Work out the finished part from the listing and answer in its coordinate system (mm). A direction names the side the tool comes from. Round coordinates to 2 decimals unless told otherwise and drop trailing zeros. Use one line per item in the form item = value. Start each with the question number.
Q1. Given P1, Ø10, axis at x = -24.5, y = -16, coming from the -Z side; P2, Ø12, axis at x = -12, z = -65.5, coming from the -Y side; P3, Ø2, axis at x = -10, z = -59, coming from the +Y side, each flat-ended and moving along its own axis, determine where each tip first touches the part or whether it passes through.
Q2. Which of the six approach directions +Z, -Z, +X, -X, +Y, -Y give full straight-line access (tool end or side, diameter ignored) to faces 3 (the cylindrical face through (-31.97, -27.64, 124.47)), 4 (the cylindrical face through (-21, 101, 0)), 5 (the flat face through (-12, 2, 101))?
Q3. The part is cut by section A-A on x = -18. State how many separate pieces and enclosed holes the cut face has, plus the area to 3 significant figures.
Q4. Find the intervals of material crossed by line 1 (Z direction, x = -24.5, y = 0); line 2 (Z direction, x = -21.75, y = -62.5); line 3 (X direction, y = -94, z = -57.5), in increasing order. Write a range as [from, to].
Q5. For a pull along Z with two mould halves and no side action, classify faces 1 (the cylindrical face through (-19.69, -107.13, 82.15)), 2 (the flat face through (-29, 125, 0)) as +Z half, -Z half, draft (parallel to the pull), parting line (faces both ways), or undercut.
from build123d import *

# Parameters (mm, degrees)
F2_R     = 6
F3_DEPTH = 30.001
F4_R     = 8.5
F5_DEPTH = 12
F6_R     = 5.25
F7_DEPTH = 24
F8_SIZE  = 2
F9_SIZE  = 1
F10_SIZE = 0.5


with BuildPart() as f1:
    # F0 (on Top) → F1 (revolve)
    with BuildSketch(Plane.XY):
        Polygon((-30, 80), (0, 80), (0, 115), (-5, 115), (-5, 135), (-35, 135), (-35, 127.5), (-30, 127.5), align=None)
    revolve(axis=Axis((-42.337157, 0, 0), (-1, 0, 0)))

    # F2 (on face) → F3 (cut, through all)
    with BuildSketch(Plane(origin=(-30, 0, 0), x_dir=(0, -1, 0), z_dir=(-1, 0, 0))):
        with Locations((-95, 0)):
            Circle(F2_R)
        with Locations((0, -95)):
            Circle(F2_R)
        with Locations((95, 0)):
            Circle(F2_R)
        with Locations((0, 95)):
            Circle(F2_R)
    extrude(amount=-F3_DEPTH, mode=Mode.SUBTRACT)

    # F4 (on face) → F5 (cut)
    with BuildSketch(Plane.YZ):
        with Locations((0, -95)):
            Circle(F4_R)
        with Locations((95, 0)):
            Circle(F4_R)
        with Locations((0, 95)):
            Circle(F4_R)
        with Locations((-95, 0)):
            Circle(F4_R)
    extrude(amount=-F5_DEPTH, mode=Mode.SUBTRACT)

    # F6 (on face) → F7 (cut)
    with BuildSketch(Plane.YZ.offset(-5)):
        with Locations((125, 0)):
            Circle(F6_R)
        with Locations((-62.5, 108.253175)):
            Circle(F6_R)
        with Locations((-62.5, -108.253175)):
            Circle(F6_R)
    extrude(amount=-F7_DEPTH, mode=Mode.SUBTRACT)

    # F8
    f8_edges = [f1.edges().sort_by_distance(p)[0] for p in [
        (-30, -80, 0),
        (-35, -135, 0),
        (0, -80, 0),
    ]]
    chamfer(f8_edges, length=F8_SIZE)

    # F9
    f9_edges = [f1.edges().sort_by_distance(p)[0] for p in [
        (-35, -127.5, 0),
        (-30, 6, -95),
        (-30, 101, 0),
        (-30, 6, 95),
        (-30, -89, 0),
        (0, -8.5, 95),
        (0, 86.5, 0),
        (0, -8.5, -95),
        (0, -103.5, 0),
        (-5, 119.75, 0),
        (-5, -67.75, 108.253175),
        (-5, -67.75, -108.253175),
        (-5, -135, 0),
    ]]
    chamfer(f9_edges, length=F9_SIZE)

    # F10
    f10_edges = [f1.edges().sort_by_distance(p)[0] for p in [
        (0, -115, 0),
    ]]
    chamfer(f10_edges, length=F10_SIZE)


solid = f1.part
Found:
q1.P1 = -134.55
q1.P2 = -121.18
q1.P3 = 121.91
q2.face_3 = -X
q2.face_4 = +X, -X
q2.face_5 = +X
q3.separate_pieces = 1
q3.enclosed_holes = 8
q3.area = 36,400 mm²
q4.line_1 = [-135, -101], [-89, -80], [80, 89], [101, 135]
q4.line_2 = [-119.66, -113.5], [-103, -49.94], [49.94, 103], [113.5, 119.66]
q4.line_3 = [-30, 0]
q5.face_1 = parting line
q5.face_2 = undercut
